Design review of the part built by this model. Coordinates are the model's own, in mm. Coordinates: 2 decimals unless noted, no trailing zeros. Loops run counter-clockwise (first coordinate to the right, second up) from the corner with the lowest first, then second, coordinate; pieces in that order, holes last. Notation, with made-up numbers: (76.25, 27.25) -> (131.25, 27.25) arc R15 cw to (131.25, 49.25) -> close; hole circle Ø8 at (2, -26). An arc over 180 degrees is marked (long way). Answer in a Markdown table with one row per item.
```python
from build123d import *

# Parameters (mm, degrees)
F0_R            = 241.3
F0_R_2          = 25.4
F1_DEPTH        = 3.175
F2_R            = 2.15265
F3_DEPTH        = 3.175
F3_COPIES_COUNT = 6
F4_R            = 2.15265
F5_DEPTH        = 3.175


# Not quite as in the source:
# - a pattern or mirror of a feature is missing from the dataset's text; its kind, count and spacing are read off the source's solid


with BuildPart() as f1:
    # F0 (on Top) → F1 (new body)
    with BuildSketch(Plane.XY):
        Circle(F0_R)
        Circle(F0_R_2, mode=Mode.SUBTRACT)
    extrude(amount=F1_DEPTH)

    # F2 (on face) → F3 (cut, through all)
    with BuildSketch(Plane.XY.offset(3.175)):
        with BuildLine():
            ThreePointArc((13.1131726267, -30.6501812378), (0, -33.3375), (-13.1131726267, -30.6501812378))
            Line((-13.1131726267, -30.6501812378), (-43.8387272582, -83.8684029504))
            ThreePointArc((-43.8387272582, -83.8684029504), (0, -94.6347875841), (43.8387272582, -83.8684029504))
            Line((43.8387272582, -83.8684029504), (13.1131726267, -30.6501812378))
        make_face()
        with BuildLine():
            Line((-82.5017818898, -150.8347779481), (-113.2273365214, -204.0529996607))
            ThreePointArc((-113.2273365214, -204.0529996607), (0, -233.3625), (113.2273365214, -204.0529996607))
            Line((113.2273365214, -204.0529996607), (82.5017818898, -150.8347779481))
            ThreePointArc((82.5017818898, -150.8347779481), (0, -171.923454635), (-82.5017818898, -150.8347779481))
        make_face()
        with BuildLine():
            ThreePointArc((47.8074772582, -90.742479593), (0, -102.5658446291), (-47.8074772582, -90.742479593))
            Line((-47.8074772582, -90.742479593), (-78.5330318898, -143.9607013056))
            ThreePointArc((-78.5330318898, -143.9607013056), (0, -163.9881721899), (78.5330318898, -143.9607013056))
            Line((78.5330318898, -143.9607013056), (47.8074772582, -90.742479593))
        make_face()
        with Locations((0, -98.6003161066)):
            Circle(F2_R)
        with Locations((0, -167.9558134125)):
            Circle(F2_R)
        with Locations((0, -237.33125)):
            Circle(F2_R)
    f3 = extrude(amount=-F3_DEPTH, mode=Mode.SUBTRACT)

    # F3_copies: F3 ×6 about axis
    f3_copies_axis = Axis((0, 0, 0), (0, 0, 1))
    for i in range(1, F3_COPIES_COUNT):
        add(f3.rotate(f3_copies_axis, i * 360 / F3_COPIES_COUNT), mode=Mode.SUBTRACT)

    # F4 (on face) → F5 (cut, through all)
    with BuildSketch(Plane.XY.offset(3.175)):
        with Locations((-20.76684228, 20.76684228)):
            Circle(F4_R)
        with Locations((20.76684228, 20.76684228)):
            Circle(F4_R)
        with Locations((20.76684228, -20.76684228)):
            Circle(F4_R)
        with Locations((-20.76684228, -20.76684228)):
            Circle(F4_R)
    extrude(amount=-F5_DEPTH, mode=Mode.SUBTRACT)


solid = f1.part
```
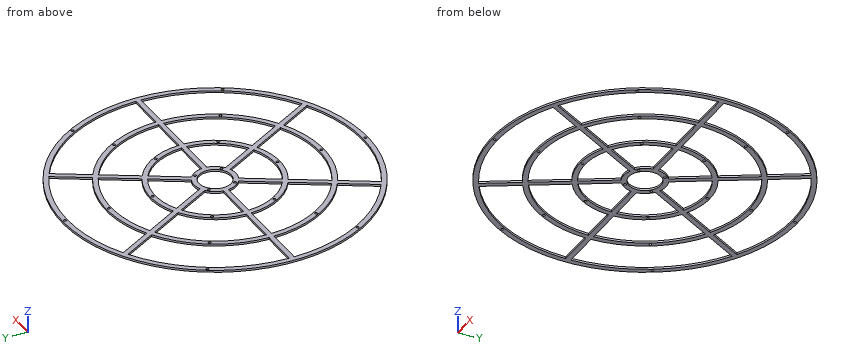
(1) To check wall thickness, follow probe 1 along X at (y, z) = (-198, 3); probe 2 along Y at (x, z) = (151.5, 0.35); probe 3 along X at (y, z) = (-183, 3). State the ranges of each line that lie inside material, in increasing order.
Evaluation:
| item | result |
|---|---|
| probe 1 | x = -137.92 to -123.51, -118.9 to -109.73, 109.73 to 118.9, 123.51 to 137.92 |
| probe 2 | y = -187.81 to -177.5, -81.27 to -62.77, -3.97 to 3.97, 62.77 to 81.27, 177.5 to 187.81 |
| probe 3 | x = -157.28 to -144.81, -110.24 to -101.07, 101.07 to 110.24, 144.81 to 157.28 |
(2) Take a section at A-A on y = -61. Count the separate pieces of the cut face and the enclosed holes in it, and give its area (3 significant figures).
Evaluation:
| item | result |
|---|---|
| separate pieces | 8 |
| enclosed holes | 0 |
| area | 229 mm² |
(3) For pin 1 (1.6 mm diameter, centred on x = 124, z = 1, fed in from -Y); pin 2 (1.5 mm diameter, centred on x = -162, z = 2.5, fed in from +Y); pin 3 (1 mm diameter, centred on x = 188, z = 1.5, fed in from +Y), all flat-tipped, find the tip position at first contact; note any pin that passes through.
Evaluation:
| item | result |
|---|---|
| pin 1 | stops at y = -207.48 |
| pin 2 | stops at y = 179.51 |
| pin 3 | stops at y = 151.89 |
(4) Take a section at B-B on x = 192. Give the boundary of the cut face in (y, z) (3 decimals), and give its area (3 significant figures).
Evaluation:
| item | result |
|---|---|
| outline | (-146.156, 0) -> (-132.643, 0) -> (-132.643, 3.175) -> (-146.156, 3.175) -> close; (-3.969, 0) -> (3.969, 0) -> (3.969, 3.175) -> (-3.969, 3.175) -> close; (132.643, 0) -> (146.156, 0) -> (146.156, 3.175) -> (132.643, 3.175) -> close |
| area | 111 mm² |
